CAD build for the part. Positions are in the model's coordinates, mm. A direction names the side the tool comes from. Round coordinates to 2 decimals unless told otherwise and drop trailing zeros. Order: outer loops, then holes, each group sorted by start corner. A loop starts at its lowest first (then second) coordinate and runs counter-clockwise, first axis right, second up. Notation, with made-up numbers: M 18.25,72.25 L 37.25,72.25 A14 cw 37.25,92.25 Z; hole C -40,20 d1. An arc over 180 degrees is marked long. Answer as a JSON object with one key per item and string values.
```python
from build123d import *

# Parameters (mm, degrees)
SKETCH1_W                = 28.18
SKETCH1_H                = 44
BOSS_EXTRUDE1_DEPTH      = 11
BOSS_EXTRUDE1_DEPTH_BACK = 2
CUT_EXTRUDE1_DEPTH       = 37
SKETCH4_W                = 20.18
SKETCH4_H                = 4
CUT_EXTRUDE2_DEPTH       = 48
CUT_EXTRUDE3_DEPTH       = 1.75
SKETCH7_R                = 1.8
CUT_EXTRUDE4_DEPTH       = 23
SKETCH10_W               = 11.795844225
SKETCH10_H               = 4.586005201
CUT_EXTRUDE7_DEPTH       = 53
FILLET1_R                = 1
SKETCH8_R                = 3.25
CUT_EXTRUDE5_DEPTH       = 1.75


with BuildPart() as part:
    # Sketch1 → Boss-Extrude1 (new body, two sides)
    with BuildSketch(Plane.XY) as boss_extrude1_sk:
        Rectangle(SKETCH1_W, SKETCH1_H)
    extrude(amount=BOSS_EXTRUDE1_DEPTH)
    extrude(boss_extrude1_sk.sketch, amount=-BOSS_EXTRUDE1_DEPTH_BACK)

    # Sketch3 → Cut-Extrude1 (cut)
    with BuildSketch(Plane.ZY.offset(14.09)):
        Polygon((8, 7.25), (11, 7.25), (11, -7.25), (8, -7.25), (8, -17.75), (3, -17.75), (3, -7.25), (1.5033938, -7.25), (1.5033938, 7.25), (3, 7.25), (3, 17.75), (8, 17.75), align=None)
    extrude(amount=-CUT_EXTRUDE1_DEPTH, mode=Mode.SUBTRACT)

    # Sketch4 → Cut-Extrude2 (cut)
    with BuildSketch(Plane.XZ.offset(22)):
        with Locations((4, 9)):
            Rectangle(SKETCH4_W, SKETCH4_H)
    extrude(amount=-CUT_EXTRUDE2_DEPTH, mode=Mode.SUBTRACT)

    # Sketch5 → Cut-Extrude3 (cut)
    with BuildSketch(Plane(origin=(0, 0, -2), x_dir=(-1, 0, 0), z_dir=(0, 0, -1))):
        with BuildLine():
            Line((-9.422350513, -22), (-5.513274624, -22))
            add(Edge.make_bspline(
                [(-14.09, 12.943541527), (17.027152303, 14.230895657), (-0.913223026, -5.637747584), (-5.513274624, -22)],
                knots=[0, 0, 0, 0, 0.88215351, 0.88215351, 0.88215351, 0.88215351], degree=3))
            Line((-14.09, 12.943541527), (-14.09, 8.727219843))
            add(Edge.make_bspline(
                [(-14.09, 8.727219843), (12.710361443, 11.678555955), (-5.250487577, -7.026945605), (-9.422350513, -22)],
                knots=[0, 0, 0, 0, 0.871233208, 0.871233208, 0.871233208, 0.871233208], degree=3))
        make_face()
        with BuildLine():
            add(Edge.make_bspline(
                [(-14.09, 3.523280295), (7.913446573, 11.6376574), (-14.09, -14.545652593)],
                knots=[0, 0, 0, 1, 1, 1], degree=2))
            Line((-14.09, 3.523280295), (-14.09, -1.131328535))
            add(Edge.make_bspline(
                [(-14.09, -1.131328535), (-1.654052468, 3.211926994), (-14.09, -7.240502624)],
                knots=[0, 0, 0, 1, 1, 1], degree=2))
            Line((-14.09, -7.240502624), (-14.09, -14.545652593))
        make_face()
        with BuildLine():
            add(Edge.make_bspline(
                [(-2.448223174, 22), (19.56705897, 11.536361781), (5.151599528, -7.62224079), (5.592236917, -22)],
                knots=[0, 0, 0, 0, 0.832841206, 0.832841206, 0.832841206, 0.832841206], degree=3))
            Line((-2.448223174, 22), (-13.413117725, 22))
            add(Edge.make_bspline(
                [(-13.413117725, 22), (18.496116363, 13.047461166), (3.546154763, -4.863207343), (0.001206333, -22)],
                knots=[0, 0, 0, 0, 0.886771983, 0.886771983, 0.886771983, 0.886771983], degree=3))
            Line((0.001206333, -22), (5.592236917, -22))
        make_face()
    extrude(amount=-CUT_EXTRUDE3_DEPTH, mode=Mode.SUBTRACT)

    # Sketch7 → Cut-Extrude4 (cut)
    with BuildSketch(Plane.XY.offset(11)):
        with Locations((-10.09, 12.4)):
            Circle(SKETCH7_R)
        with Locations((-10.09, -12.4)):
            Circle(SKETCH7_R)
    extrude(amount=-CUT_EXTRUDE4_DEPTH, mode=Mode.SUBTRACT)

    # Sketch10 → Cut-Extrude7 (cut)
    with BuildSketch(Plane(origin=(0, 22, 0), x_dir=(1, 0, 0), z_dir=(0, 1, 0))):
        with Locations((-10.712086776, -9.2930026)):
            Rectangle(SKETCH10_W, SKETCH10_H)
    extrude(amount=-CUT_EXTRUDE7_DEPTH, mode=Mode.SUBTRACT)

    # Fillet1
    fillet1_edges = [part.edges().sort_by_distance(p)[0] for p in [
        (-14.09, 17.75, 5),
        (14.09, -12.5, 3),
        (14.09, 12.5, 3),
        (14.09, 17.75, 5),
        (0, -17.75, 3),
        (0, 17.75, 3),
        (-14.09, -12.5, 3),
        (-14.09, -17.75, 5),
        (-14.09, 12.5, 3),
        (14.09, -17.75, 5),
        (0, -17.75, 7),
        (0, 17.75, 7),
    ]]
    fillet(fillet1_edges, radius=FILLET1_R)

    # Sketch8 → Cut-Extrude5 (cut)
    with BuildSketch(Plane(origin=(0, 0, -2), x_dir=(-1, 0, 0), z_dir=(0, 0, -1))):
        with Locations((10.09, -12.4)):
            Circle(SKETCH8_R)
        with Locations((10.09, 12.4)):
            Circle(SKETCH8_R)
    extrude(amount=-CUT_EXTRUDE5_DEPTH, mode=Mode.SUBTRACT)


solid = part.part
```
Item 1: Drop flat-ended pins along their axis: pin 1 Ø3 at (x, y) = (-1.5, -13) entering from +Z; pin 2 Ø2 at (x, y) = (3, -6) entering from +Z; pin 3 Ø1 at (y, z) = (6, 4) entering from -X. Give the stop position or say it passes through.
Worked answers:
{"pin 1": "stops at z = 3", "pin 2": "stops at z = 1.5", "pin 3": "passes through"}
Item 2: Saw through at A-A on z = 1. List the corners of the cut face in (x, y), and give its area (3 significant figures).
Worked answers:
{"outline": "M -14.09,-22 L 14.09,-22 L 14.09,22 L -14.09,22 Z; hole C -10.09,-12.4 d3.6; hole C -10.09,12.4 d3.6", "area": "1,220 mm2"}
Item 3: Saw through at B-B on z = -1. State how many separate pieces and enclosed holes the cut face has, and give its area (3 significant figures).
Worked answers:
{"separate pieces": "4", "enclosed holes": "0", "area": "704 mm2"}
Item 4: Wall check: line 1 along Y through (x, z) = (-10.25, -1.5); line 2 along Y through (x, z) = (-10.09, 1.75); line 3 along Y through (x, z) = (1.5, 2). Give the ranges that are in metal, low to high. Write a range as [from, to].
Worked answers:
{"line 1": "y = [-22, -15.65], [-9.15, 9.15], [15.65, 22]", "line 2": "y = [-22, -14.2], [-10.6, -7.25], [7.25, 10.6], [14.2, 22]", "line 3": "y = [-22, -7.25], [7.25, 22]"}
Item 5: Two-plate mould, pull along Y, no slides. Class faces 6 (the flat face through (0, -17.75, 5)), 7 (the flat face through (0, -22, 3)), 8 (the flat face through (6.6, -5.1, -2)): released by +Y, released by -Y, zero draft, split by the parting line, or undercut.
Worked answers:
{"face 6": "undercut", "face 7": "released by -Y", "face 8": "zero draft"}
Item 6: 3-axis set-ups, long thin cutter, end or side, ignore diameter. For faces 1 (the cylindrical face through (-13.805, -11.933, 2.699)), 2 (the cylindrical face through (13.805, -18.051, 5.521)), 3 (the cylindrical face through (0.183, -17.449, 3.285)), 4 (the cylindrical face through (-13.224, -13.26, -1.137)), 5 (the flat face through (0, -20, 7)): which of +Z, -Z, +X, -X, +Y, -Y reach the whole face in a straight line?
Worked answers:
{"face 1": "+Z, -X", "face 2": "+Z, +X", "face 3": "+Z, +X, -X", "face 4": "-Z", "face 5": "+Z, +X, -X, +Y, -Y"}
